from build123d import *

# Parameters (mm, degrees)
SKETCH_1_R      = 12
SKETCH_1_R_2    = 1.7
SKETCH_1_R_3    = 2.1
SKETCH_1_W      = 42
SKETCH_1_H      = 22
EXTRUDE_1_DEPTH = 3
FILLET_1_R      = 12


with BuildPart() as part:
    # 草图1 → 凸台-拉伸1 (new body)
    with BuildSketch(Plane(origin=(0, 0, 0), x_dir=(1, 0, 0), z_dir=(0, 1, 0))):
        with BuildLine():
            Line((0, -26), (95, -26))
            Line((95, -26), (95, 26))
            Line((95, 26), (0, 26))
            ThreePointArc((0, 26), (-26, 0), (0, -26))
        make_face()
        with Locations(Location((0, 0, 0), (0, 0, 270))):
            Circle(SKETCH_1_R, mode=Mode.SUBTRACT)
        with Locations(Location((0, -21, 0), (0, 0, 270))):
            Circle(SKETCH_1_R_2, mode=Mode.SUBTRACT)
        with Locations(Location((35.5, 5, 0), (0, 0, 270))):
            Circle(SKETCH_1_R_3, mode=Mode.SUBTRACT)
        with Locations(Location((35.5, -5, 0), (0, 0, 270))):
            Circle(SKETCH_1_R_3, mode=Mode.SUBTRACT)
        with Locations(Location((84.5, -5, 0), (0, 0, 90))):
            Circle(SKETCH_1_R_3, mode=Mode.SUBTRACT)
        with Locations(Location((84.5, 5, 0), (0, 0, 90))):
            Circle(SKETCH_1_R_3, mode=Mode.SUBTRACT)
        with Locations(Location((-18.186533479, -10.5, 0), (0, 0, 270))):
            Circle(SKETCH_1_R_2, mode=Mode.SUBTRACT)
        with Locations(Location((-18.186533479, 10.5, 0), (0, 0, 270))):
            Circle(SKETCH_1_R_2, mode=Mode.SUBTRACT)
        with Locations(Location((0, 21, 0), (0, 0, 270))):
            Circle(SKETCH_1_R_2, mode=Mode.SUBTRACT)
        with Locations(Location((18.186533479, 10.5, 0), (0, 0, 270))):
            Circle(SKETCH_1_R_2, mode=Mode.SUBTRACT)
        with Locations(Location((18.186533479, -10.5, 0), (0, 0, 270))):
            Circle(SKETCH_1_R_2, mode=Mode.SUBTRACT)
        with Locations((60, 0)):
            Rectangle(SKETCH_1_W, SKETCH_1_H, mode=Mode.SUBTRACT)
    extrude(amount=EXTRUDE_1_DEPTH)

    # 圆角1
    fillet_1_edges = [part.edges().sort_by_distance(p)[0] for p in [
        (95, 1.5, -26),
        (95, 1.5, 26),
    ]]
    fillet(fillet_1_edges, radius=FILLET_1_R)


solid = part.part
Geometry check sheet. Reference: the model listing, model coordinates, mm. A direction names the side the tool comes from. Give positions to 0.01 mm unless a question says otherwise; leave off trailing zeros. Order: outer loops, then holes, each group sorted by start corner. A loop starts at its lowest first (then second) coordinate and runs counter-clockwise, first axis right, second up. Notation, with made-up numbers: M 26,23 L 77,23 A18 cw 77,39 Z; hole C -36,-38.75 d1. An arc over 180 degrees is marked long. Use a Markdown table: item, result.
Item 1: Tool access check on faces 1 (the flat face through (81, 1, 0)), 2 (the flat face through (41, 1, 26)). Record the directions out of +Z, -Z, +X, -X, +Y, -Y that give a thin tool (end or side, any length) a straight path to the whole face; none if there is none.
Answers follow:
| item | result |
|---|---|
| face 1 | +Y, -Y |
| face 2 | +Z, +X, -X, +Y, -Y |
Item 2: Draft check along X on faces 3 (the flat face through (60, 1, 11)), 4 (the flat face through (34, 0, 0)), 5 (the cylindrical face through (91.39, 1.52, 22.58)). Enter one of: +X half, -X half, draft (parallel to the pull), parting line (faces both ways), or undercut.
Answers follow:
| item | result |
|---|---|
| face 3 | undercut |
| face 4 | draft |
| face 5 | +X half |
Item 3: Section check A-A (z = 0). Record the cut outline in (x, y), and give its area (3 significant figures).
Answers follow:
| item | result |
|---|---|
| outline | M -26,0 L -12,0 L -12,3 L -26,3 Z; M 12,0 L 39,0 L 39,3 L 12,3 Z; M 81,0 L 95,0 L 95,3 L 81,3 Z |
| area | 165 mm2 |
Item 4: Section check C-C (z = -21). Record the cut outline in (x, y).
Answers follow:
| item | result |
|---|---|
| outline | M -15.33,0 L -1.7,0 L -1.7,3 L -15.33,3 Z; M 1.7,0 L 92.75,0 L 92.75,3 L 1.7,3 Z |
Item 5: Depth check by flat-ended pin: P1, Ø2.5, axis at x = 84.5, z = 5, coming from the +Y side. Enter the tip coordinate at first touch or a pass-through.
Answers follow:
| item | result |
|---|---|
| P1 | passes through |
Item 6: Material ranges on line 1 along Z through (x, y) = (47, 0.7); line 2 along X through (y, z) = (1.9, -5); line 3 along Z through (x, y) = (-17, 2.3), recorded low to high.
Answers follow:
| item | result |
|---|---|
| line 1 | z = -26 to -11, 11 to 26 |
| line 2 | x = -25.51 to -10.91, 10.91 to 33.4, 37.6 to 39, 81 to 82.4, 86.6 to 95 |
| line 3 | z = -19.67 to -11.72, -9.28 to 9.28, 11.72 to 19.67 |
Item 7: Section check D-D (y = 1.45). State how many separate pieces and enclosed holes the cut face has, and give its area (3 significant figures).
Answers follow:
| item | result |
|---|---|
| separate pieces | 1 |
| enclosed holes | 12 |
| area | 4,450 mm2 |
Item 8: Section check B-B (x = 6.5). Record the cut outline in (y, z).
Answers follow:
| item | result |
|---|---|
| outline | M 0,-26 L 3,-26 L 3,-10.09 L 0,-10.09 Z; M 0,10.09 L 3,10.09 L 3,26 L 0,26 Z |
